Part print with two shaded views. Sizes in mm from the minimum x, y, z corner. A direction names the side the tool comes from. Round coordinates to 2 decimals unless told otherwise and drop trailing zeros. Write each loop counter-clockwise with the first axis right and the second up, starting at its lowest first coordinate (ties: lowest second). Pieces come first, ordered by that corner, then holes. Notation, with made-up numbers: (-14.75, 26) -> (37.25, 26) arc R13 cw to (37.25, 45) -> close; hole circle Ø8 at (-32, 56). An arc over 180 degrees is marked (long way). Return JSON: item names as keys, results as strings. Group by question number.
(1) Drop flat-ended pins along their axis: pin 1 Ø1.5 at (x, y) = (14, 8.5) entering from -Z; pin 2 Ø10 at (y, z) = (11.5, 62.5) entering from -X; pin 3 Ø6 at (y, z) = (26, 66) entering from +X. Give the stop position or say it passes through.
(2) Drill centre lines: L1, parallel to Z at x = 4.5, y = 14; L2, parallel to Y at x = 18.5, z = 51.5; L3, parallel to X at y = 14.75, z = 64 (1 decimal). Where is each one in solid material? Low to high. Write a range as from..to.
(3) Saw through at A-A (y = 15). List the corners of the cut face in (x, z), plus the area to 3 significant figures.
(4) Saw through at C-C (z = 51.5). List the corners of the cut face in (x, y).
(5) Saw through at B-B (x = 19.5). List the corners of the cut face in (y, z).
(6) Tool access for the marked faces 1 and 2: list every direction of +Z, -Z, +X, -X, +Y, -Y with a clear straight run to the whole face (end or side of a thin tool).
(7) Saw through at D-D (y = 27.5). List the corners of the cut face in (x, z).
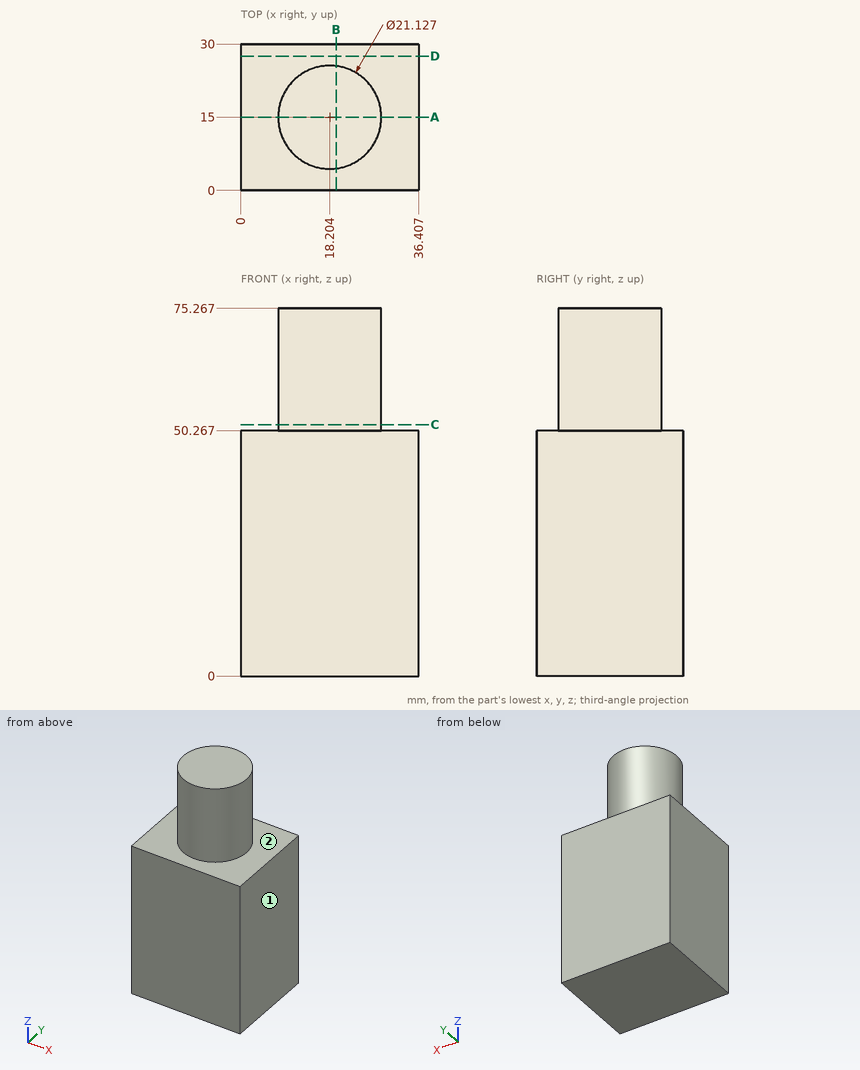
Computed values:
{
 "1": {"pin 1": "z = 0", "pin 2": "x = 7.64", "pin 3": "x = 25.1"},
 "2": {"L1": "0..50.27", "L2": "4.44..25.56", "L3": "7.6..28.8"},
 "3": {"outline": "(0, 0) -> (36.41, 0) -> (36.41, 50.27) -> (28.77, 50.27) -> (28.77, 75.27) -> (7.64, 75.27) -> (7.64, 50.27) -> (0, 50.27) -> close", "area": "2,360 mm2"},
 "4": {"outline": "circle Ø21.13 at (18.2, 15)"},
 "5": {"outline": "(0, 0) -> (30, 0) -> (30, 50.27) -> (25.48, 50.27) -> (25.48, 75.27) -> (4.52, 75.27) -> (4.52, 50.27) -> (0, 50.27) -> close"},
 "6": {"face 1": "+Z, -Z, +X, +Y, -Y", "face 2": "+Z"},
 "7": {"outline": "(0, 0) -> (36.41, 0) -> (36.41, 50.27) -> (0, 50.27) -> close"}
}
